Check sheet for the modelled part. Datum: model origin and axes. Units: mm. A direction names the side the tool comes from. Coordinates: 2 decimals unless noted, no trailing zeros. Write each loop counter-clockwise with the first axis right and the second up, starting at its lowest first coordinate (ties: lowest second). Pieces come first, ordered by that corner, then holes. Notation, with made-up numbers: M -1.5,66 L 57.5,66 A16 cw 57.5,71 Z; hole C 10.5,46 d7. An arc over 180 degrees is marked long. Answer as CSV lines item,"result". Start each with the question number.
Q1. Access from +Z, -Z, +X, -X, +Y, -Y to the whole of each face (thin tool, end or side, straight path). Record for faces 1 (the flat face through (36, -32, 51.789)), 2 (the cylindrical face through (2.865, -3.803, -73.396)), 3 (the flat face through (18, -32, 81.789)).
Q2. Depth check by flat-ended pin: pin 1 Ø8 at (y, z) = (-28, 58) entering from +X; pin 2 Ø25 at (y, z) = (-34, -9.5) entering from -X; pin 3 Ø12 at (x, y) = (-18.5, -10) entering from +Z. Enter the tip coordinate at first touch or a pass-through.
Q3. Sectioned sample at C-C, the plane x = -7.5. Record the cut outline in (y, z).
Q4. Mould release check, pull along X, two halves, no side actions. Record for faces 4 (the flat face through (-16.065, -32.045, -79.511)), 5 (the flat face through (36, -32, -78.211)), 6 (the cylindrical face through (2.865, -61.302, -73.396)): pulls with the +X half, pulls with the -X half, needs draft (parallel to the pull), parting line crosses it, or undercut.
Q5. Thickness scan on line 1 along Z through (x, y) = (33.5, -52); line 2 along Y through (x, z) = (-19, -62); line 3 along Z through (x, y) = (26.5, -31). Record the ranges inside material, lowest first. Write a range as from..to.
Q6. Sectioned sample at A-A, the plane z = 14. Record the cut outline in (x, y), then the cut area to 4 significant figures.
Q7. Sectioned sample at B-B, the plane y = -17.5. Count the separate pieces of the cut face and the enclosed holes in it, then the cut area to 3 significant figures.
from build123d import *

# Parameters (mm, degrees)
PAD_DEPTH              = 65
POCKET_DEPTH           = 65.001
SKETCH002_R            = 4
POCKET001_DEPTH        = 65.001
LINEARPATTERN_COUNT    = 6
LINEARPATTERN_PITCH    = 29
SKETCH003_W            = 160
SKETCH003_H            = 50
POCKET002_DEPTH        = 55
SKETCH004_W            = 30
SKETCH004_H            = 65
POCKET003_DEPTH        = 5
SKETCH005_R            = 3
POCKET004_DEPTH        = 12.172573
SKETCH035_R            = 10
POCKET023_DEPTH        = 65.001
LINEARPATTERN001_COUNT = 3
LINEARPATTERN001_PITCH = 32.5
SKETCH076_W            = 10
SKETCH076_H            = 65
POCKET047_DEPTH        = 1


with BuildPart() as part:
    # Sketch → Pad (new body)
    with BuildSketch(Plane.XZ):
        Polygon((-2.003095, 92.602939), (37.996905, 92.602939), (37.996905, -82.397061), (-12.003095, -82.397061), (-27.003095, -71.740207), (-27.003095, 73.259793), align=None)
    extrude(amount=PAD_DEPTH)

    # Sketch001 (on Face8 of Pad) → Pocket (cut, through all)
    with BuildSketch(Plane.XZ.offset(65)):
        with BuildLine():
            ThreePointArc((8.996905, 77.602939), (2.996905, 83.602939), (-3.003095, 77.602939))
            Line((-3.003095, 77.602939), (-3.003095, -67.397061))
            ThreePointArc((-3.003095, -67.397061), (2.996905, -73.397061), (8.996905, -67.397061))
            Line((8.996905, 77.602939), (8.996905, -67.397061))
        make_face()
    extrude(amount=-POCKET_DEPTH, mode=Mode.SUBTRACT)

    # Sketch002 (on Face5 of Pocket) → Pocket001 (cut, through all)
    with BuildSketch(Plane.XZ.offset(65)):
        with Locations((17.996905, 77.602939)):
            Circle(SKETCH002_R)
    pocket001 = extrude(amount=-POCKET001_DEPTH, mode=Mode.SUBTRACT)

    # LinearPattern: Pocket001 ×6
    with Locations(*[(0, 0, -i * LINEARPATTERN_PITCH) for i in range(1, LINEARPATTERN_COUNT)]):
        add(pocket001, mode=Mode.SUBTRACT)

    # Sketch003 (on Face1 of LinearPattern) → Pocket002 (cut)
    with BuildSketch(Plane(origin=(-27.003095, 0, 0), x_dir=(0, 0, -1), z_dir=(-1, 0, 0))):
        with Locations((-1.789118, 32.5)):
            Rectangle(SKETCH003_W, SKETCH003_H)
    extrude(amount=-POCKET002_DEPTH, mode=Mode.SUBTRACT)

    # Sketch004 (on Face8 of Pocket002) → Pocket003 (cut)
    with BuildSketch(Plane(origin=(37.996905, 0, 0), x_dir=(0, 0, 1), z_dir=(1, 0, 0))):
        with Locations((-63.210882, 32.5)):
            Rectangle(SKETCH004_W, SKETCH004_H)
        with Locations((66.789118, 32.5)):
            Rectangle(SKETCH004_W, SKETCH004_H)
    extrude(amount=-POCKET003_DEPTH, mode=Mode.SUBTRACT)

    # Sketch005 → Pocket004 (cut, through all)
    with BuildSketch(Plane(origin=(25.825332, 0, 0), x_dir=(0, 0, 1), z_dir=(1, 0, 0))):
        with Locations((-63.210882, 17.5)):
            Circle(SKETCH005_R)
        with Locations((-63.210882, 47.5)):
            Circle(SKETCH005_R)
        with Locations((66.789118, 47.5)):
            Circle(SKETCH005_R)
        with Locations((66.789118, 17.5)):
            Circle(SKETCH005_R)
    extrude(amount=POCKET004_DEPTH, mode=Mode.SUBTRACT)

    # Sketch035 → Pocket023 (cut, through all)
    with BuildSketch(Plane(origin=(37.996905, 0, 0), x_dir=(0, 0, 1), z_dir=(1, 0, 0))):
        with Locations((-31.789585, 32.5)):
            Circle(SKETCH035_R)
    pocket023 = extrude(amount=-POCKET023_DEPTH, mode=Mode.SUBTRACT)

    # LinearPattern001: Pocket023 ×3
    with Locations(*[(0, 0, i * LINEARPATTERN001_PITCH) for i in range(1, LINEARPATTERN001_COUNT)]):
        add(pocket023, mode=Mode.SUBTRACT)

    # Sketch076 (on Face13 of Pocket004) → Pocket047 (cut)
    with BuildSketch(Plane(origin=(32.996905, 0, 0), x_dir=(0, 0, 1), z_dir=(1, 0, 0))):
        with Locations((-63.210882, 32.5)):
            Rectangle(SKETCH076_W, SKETCH076_H)
        with Locations((66.789118, 32.5)):
            Rectangle(SKETCH076_W, SKETCH076_H)
    extrude(amount=-POCKET047_DEPTH, mode=Mode.SUBTRACT)


solid = part.part
Output:
1,face 1,"+X, +Y, -Y"
1,face 2,"+Y, -Y"
1,face 3,"-X"
2,pin 1,"stops at x = 33"
2,pin 2,"stops at x = 28"
2,pin 3,"stops at z = 84.48"
3,outline,"M -65,-82.4 L 0,-82.4 L 0,88.35 L -65,88.35 Z; hole M -57.5,-78.21 L -7.5,-78.21 L -7.5,81.79 L -57.5,81.79 Z"
4,face 4,"pulls with the -X half"
4,face 5,"needs draft"
4,face 6,"undercut"
5,line 1,"z = -82.4..-78.21, -48.21..51.79, 81.79..92.6"
5,line 2,"y = -65..-57.5, -7.5..0"
5,line 3,"z = -82.4..-78.21, 81.79..92.6"
6,outline,"M -27,-65 L -3,-65 L -3,-57.5 L -27,-57.5 Z; M -27,-7.5 L -3,-7.5 L -3,0 L -27,0 Z; M 9,-65 L 38,-65 L 38,0 L 9,0 L 9,-7.5 L 28,-7.5 L 28,-57.5 L 9,-57.5 Z"
6,area,"1,295 mm^2"
7,separate pieces,"3"
7,enclosed holes,"0"
7,area,"1,950 mm^2"
